Part model, mm, in its own coordinate system. A direction names the side the tool comes from. Coordinates: 2 decimals unless noted, no trailing zeros. Loops run counter-clockwise (first coordinate to the right, second up) from the corner with the lowest first, then second, coordinate; pieces in that order, holes last. Notation, with made-up numbers: M -4.75,70 L 48.25,70 A24 cw 48.25,106 Z; hole C 85,-37 d10. An arc over 180 degrees is marked long. Use a Markdown table: item, result. Add a question column.
1) Band-saw the part on B-B (x = 5). List the corners of the cut face in (y, z), plus the area to 3 significant figures.
2) Wall check: probe 1 along Z at (x, y) = (15, -63.75); probe 2 along Y at (x, z) = (5, 7.75); probe 3 along Y at (x, z) = (18.85, 17). Give the ranges that are in metal, low to high. Write a range as from..to.
3) Pin check, flat tips, straight feed: pin 1 Ø1.8 at (y, z) = (-68, 17) entering from -X; pin 2 Ø1.8 at (y, z) = (-68, 4) entering from +X; pin 3 Ø8 at (x, z) = (17.5, 9) entering from +Y. Stop position of each tip, or through.
4) Band-saw the part on A-A (z = 17). List the corners of the cut face in (x, y).
5) Band-saw the part on D-D (z = 4). List the corners of the cut face in (x, y).
6) Pull direction Y, two halves, no side cores. Call faces 1 (the cylindrical face through (5.65, -72.07, 10.14)), 2 (the flat face through (10, -80, 10)), 3 (the flat face through (10, -28, 10)), 4 (the cylindrical face through (17.04, -69.01, 15.89)): released by +Y, released by -Y, zero draft, split by the parting line, or undercut.
7) Tool access for faces 5 (the flat face through (18.4, -56, 10.1)), 6 (the flat face through (12, -68, 15)), 7 (the cylindrical face through (18.24, -69.01, 2.89)), 8 (the flat face through (8, -48, 0)), 9 (the flat face through (17, -68, 20)): list every direction of +Z, -Z, +X, -X, +Y, -Y with a clear straight run to the whole face (end or side of a thin tool).
8) Band-saw the part on C-C (y = -57). List the corners of the cut face in (x, z).
from build123d import *

# Parameters (mm, degrees)
SKETCH_W        = 20
SKETCH_H        = 20
PAD_DEPTH       = 80
SKETCH001_R     = 3
POCKET_DEPTH    = 20.001
SKETCH002_W     = 10
SKETCH002_H     = 56
POCKET001_DEPTH = 20.001
SKETCH003_R     = 3
SKETCH003_R_2   = 1.55
POCKET002_DEPTH = 80.001
SKETCH004_W     = 2
SKETCH004_H     = 24
POCKET003_DEPTH = 10
SKETCH005_R     = 1.5
POCKET004_DEPTH = 5
SKETCH006_R     = 1.5
POCKET005_DEPTH = 20.001


with BuildPart() as part:
    # Sketch → Pad (new body)
    with BuildSketch(Plane.XZ):
        with Locations((10, 10)):
            Rectangle(SKETCH_W, SKETCH_H)
    extrude(amount=PAD_DEPTH)

    # Sketch001 (on Face3 of Pad) → Pocket (cut, through all)
    with BuildSketch(Plane(origin=(0, 0, 20), x_dir=(-1, 0, 0), z_dir=(0, 0, 1))):
        with Locations((-5, 5)):
            Circle(SKETCH001_R)
        with Locations((-5, 75)):
            Circle(SKETCH001_R)
    extrude(amount=-POCKET_DEPTH, mode=Mode.SUBTRACT)

    # Sketch002 (on Face8 of Pocket) → Pocket001 (cut, through all)
    with BuildSketch(Plane(origin=(0, 0, 20), x_dir=(-1, 0, 0), z_dir=(0, 0, 1))):
        with Locations((-15, 28)):
            Rectangle(SKETCH002_W, SKETCH002_H)
    extrude(amount=-POCKET001_DEPTH, mode=Mode.SUBTRACT)

    # Sketch003 (on Face6 of Pocket001) → Pocket002 (cut, through all)
    with BuildSketch(Plane.XZ.offset(80)):
        with Locations((15, 10)):
            Circle(SKETCH003_R)
        with Locations((15, 4)):
            Circle(SKETCH003_R_2)
    extrude(amount=-POCKET002_DEPTH, mode=Mode.SUBTRACT)

    # Sketch004 (on Face10 of Pocket002) → Pocket003 (cut)
    with BuildSketch(Plane(origin=(0, 0, 20), x_dir=(-1, 0, 0), z_dir=(0, 0, 1))):
        with Locations((-13, 68)):
            Rectangle(SKETCH004_W, SKETCH004_H)
    extrude(amount=-POCKET003_DEPTH, mode=Mode.SUBTRACT)

    # Sketch005 (on Face5 of Pocket003) → Pocket004 (cut)
    with BuildSketch(Plane(origin=(20, 0, 0), x_dir=(0, 0, 1), z_dir=(1, 0, 0))):
        with Locations((4, 68)):
            Circle(SKETCH005_R)
    extrude(amount=-POCKET004_DEPTH, mode=Mode.SUBTRACT)

    # Sketch006 (on Face5 of Pocket004) → Pocket005 (cut, through all)
    with BuildSketch(Plane(origin=(20, 0, 0), x_dir=(0, 0, 1), z_dir=(1, 0, 0))):
        with Locations((17, 68)):
            Circle(SKETCH006_R)
    extrude(amount=-POCKET005_DEPTH, mode=Mode.SUBTRACT)


solid = part.part
Entries:
| question | item | result |
|---|---|---|
| 1 | outline | M -80,0 L -78,0 L -78,20 L -80,20 Z; M -72,0 L -8,0 L -8,20 L -72,20 Z; M -2,0 L 0,0 L 0,20 L -2,20 Z; hole C -68,17 d3 |
| 1 | area | 1,350 mm2 |
| 2 | probe 1 | 0..2.45, 5.55..7, 13..20 |
| 2 | probe 2 | -80..-78, -72..-8, -2..0 |
| 2 | probe 3 | -80..-69.5, -66.5..-56 |
| 3 | pin 1 | through |
| 3 | pin 2 | x = 13.74 |
| 3 | pin 3 | y = -56 |
| 4 | outline | M 0,-80 L 12,-80 L 12,-69.5 L 0,-69.5 Z; M 0,-66.5 L 12,-66.5 L 12,-56 L 10,-56 L 10,0 L 0,0 Z; M 14,-80 L 20,-80 L 20,-69.5 L 14,-69.5 Z; M 14,-66.5 L 20,-66.5 L 20,-56 L 14,-56 Z; hole C 5,-75 d6; hole C 5,-5 d6 |
| 5 | outline | M 0,-80 L 13.45,-80 L 13.45,-56 L 10,-56 L 10,0 L 0,0 Z; M 16.55,-80 L 20,-80 L 20,-69.5 L 16.55,-69.5 Z; M 16.55,-66.5 L 20,-66.5 L 20,-56 L 16.55,-56 Z; hole C 5,-75 d6; hole C 5,-5 d6 |
| 6 | face 1 | undercut |
| 6 | face 2 | released by -Y |
| 6 | face 3 | zero draft |
| 6 | face 4 | undercut |
| 7 | face 5 | +Z, -Z, +X, +Y |
| 7 | face 6 | +Z, +Y, -Y |
| 7 | face 7 | +X |
| 7 | face 8 | -Z, +X, -X, +Y, -Y |
| 7 | face 9 | +Z, +X, -X, +Y, -Y |
| 8 | outline | M 0,0 L 20,0 L 20,20 L 14,20 L 14,12.83 A3 cw long 12,10 L 12,20 L 0,20 Z; hole C 15,4 d3.1 |
